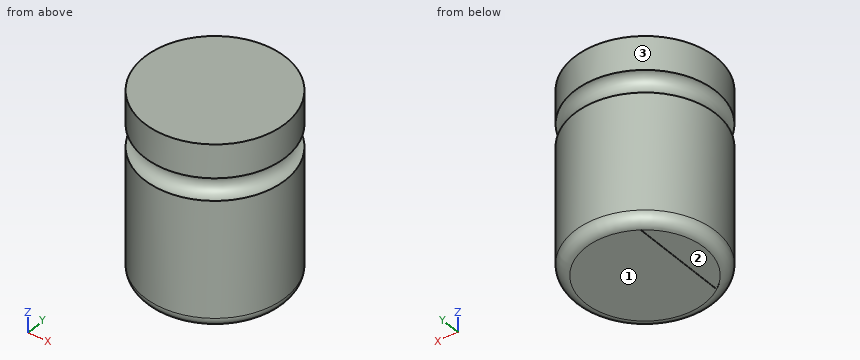
from build123d import *

# Parameters (mm, degrees)
CUT_EXTRUDE1_DEPTH = 0.01


with BuildPart() as part:
    # Sketch1 → Revolve1 (revolve)
    with BuildSketch(Plane(origin=(0, 0, 0), x_dir=(1, 0, 0), z_dir=(0, 1, 0))):
        with BuildLine():
            Line((0, 0), (3.15, 0))
            Line((3.15, 0), (3.15, 1.5))
            ThreePointArc((3.15, 1.5), (2.65, 2), (3.15, 2.5))
            Line((3.15, 2.5), (3.15, 7.7))
            ThreePointArc((3.15, 7.7), (3.003553391, 8.053553391), (2.65, 8.2))
            Line((2.65, 8.2), (0, 8.2))
            Line((0, 8.2), (0, 0))
        make_face()
    revolve(axis=Axis((0, 0, 0), (0, 0, -1)))

    # Sketch2 → Cut-Extrude1 (cut)
    with BuildSketch(Plane(origin=(0, 0, -8.2), x_dir=(-1, 0, 0), z_dir=(0, 0, -1))):
        with BuildLine():
            Line((1.5, 2.184605227), (1.5, -2.184605227))
            ThreePointArc((1.5, -2.184605227), (2.65, 0), (1.5, 2.184605227))
        make_face()
    extrude(amount=-CUT_EXTRUDE1_DEPTH, mode=Mode.SUBTRACT)


solid = part.part
The listing builds one solid part. Answer for the finished solid, in the listing's coordinates (mm). Face numbers are marked on the shaded views. Coordinates: 2 decimals unless noted, no trailing zeros. Loops run counter-clockwise (first coordinate to the right, second up) from the corner with the lowest first, then second, coordinate; pieces in that order, holes last. Notation, with made-up numbers: (26.5, 51.25) -> (84.5, 51.25) arc R27 cw to (84.5, 76.25) -> close; hole circle Ø6 at (18.25, 64). An arc over 180 degrees is marked (long way). Answer in a Markdown table with one row per item. Add a question column.
1. Determine the mould class of the marked faces 1, 2 and 3 for opening direction X: +X half, -X half, draft (parallel to the pull), parting line (faces both ways), or undercut.
2. The part is cut by section D-D, the plane z = -2.25. Write down the section's boundary in (x, y).
3. The part is cut by section C-C, the plane z = -4. Write down the section's boundary in (x, y).
4. A flat-ended cylindrical pin translates along its axis: P1, Ø1.5, axis at y = -1.5, z = -3, coming from the -X side. Find the tip coordinate at first contact, or state that the pin passes through.
5. The part is cut by section A-A, the plane x = 0. Write down the section's boundary in (y, z), then the cut area to 3 significant figures.
6. Consider line 1 (Z direction, x = -2, y = 1); line 2 (Z direction, x = -2, y = -2); line 3 (Y direction, x = 2, z = -0.5). Determine where each line is inside the solid, lowest interval first. Write a range as [from, to].
Answer below:
| question | item | result |
|---|---|---|
| 1 | face 1 | draft |
| 1 | face 2 | undercut |
| 1 | face 3 | parting line |
| 2 | outline | circle Ø5.43 at (0, 0) |
| 3 | outline | circle Ø6.3 at (0, 0) |
| 4 | P1 | x = -3.06 |
| 5 | outline | (-3.15, -7.7) arc R0.5 ccw to (-2.65, -8.2) -> (2.65, -8.2) arc R0.5 ccw to (3.15, -7.7) -> (3.15, -2.5) arc R0.5 cw to (3.15, -1.5) -> (3.15, 0) -> (-3.15, 0) -> (-3.15, -1.5) arc R0.5 cw to (-3.15, -2.5) -> close |
| 5 | area | 50.8 mm2 |
| 6 | line 1 | [-8.19, 0] |
| 6 | line 2 | [-8.17, -2.38], [-1.62, 0] |
| 6 | line 3 | [-2.43, 2.43] |
